The figure shows three views and two pictorial views of one solid part (mm, origin at its lowest corner). Answer the questions. A direction names the side the tool comes from. Round coordinates to 2 decimals unless told otherwise and drop trailing zeros. Write each loop counter-clockwise with the first axis right and the second up, starting at its lowest first coordinate (ties: lowest second). Pieces come first, ordered by that corner, then holes. Notation, with made-up numbers: M 51.5,7.5 L 65.5,7.5 A11 cw 65.5,22.5 Z; hole C -19.5,-4.5 d11. An arc over 180 degrees is marked long. Answer in a Markdown table with one row per item.
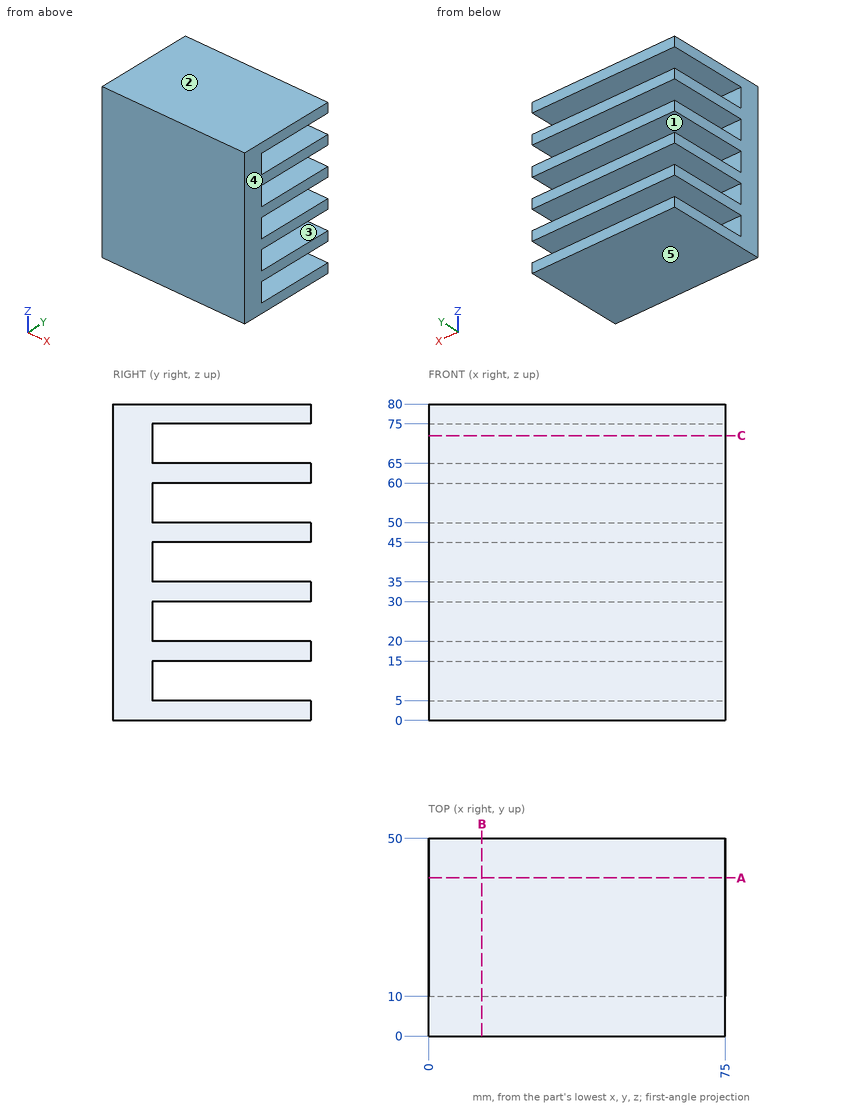
1. A tool of negligible diameter and unlimited length cuts with its end or side. For the marked faces 1 and 2, from which of +Z, -Z, +X, -X, +Y, -Y can it reach the whole face along a straight path? Write none if from no direction.
Calculated:
| item | result |
|---|---|
| face 1 | +X, -X, +Y |
| face 2 | +Z, +X, -X, +Y, -Y |
2. The part is cut by section B-B (x = 13.5). Determine the outline of the cut face in (y, z), plus the area to 3 significant figures.
Calculated:
| item | result |
|---|---|
| outline | M 0,0 L 50,0 L 50,5 L 10,5 L 10,15 L 50,15 L 50,20 L 10,20 L 10,30 L 50,30 L 50,35 L 10,35 L 10,45 L 50,45 L 50,50 L 10,50 L 10,60 L 50,60 L 50,65 L 10,65 L 10,75 L 50,75 L 50,80 L 0,80 Z |
| area | 2,000 mm² |
3. The part is cut by section C-C (z = 72). Determine the outline of the cut face in (x, y), plus the area to 3 significant figures.
Calculated:
| item | result |
|---|---|
| outline | M 0,0 L 75,0 L 75,10 L 0,10 Z |
| area | 750 mm² |
4. Determine the mould class of the marked faces 3, 4 and 5 for opening direction Z: released by +Z, released by -Z, zero draft, split by the parting line, or undercut.
Calculated:
| item | result |
|---|---|
| face 3 | undercut |
| face 4 | zero draft |
| face 5 | released by -Z |
5. Given pin 1 (8 mm diameter, centred on x = 49, z = 54.5, fed in from +Y); pin 2 (4 mm diameter, centred on x = 51.5, z = 43.5, fed in from -Y); pin 3 (1.5 mm diameter, centred on y = 15, z = 51, fed in from -X), each flat-ended and moving along its own axis, determine where each tip first touches the part or whether it passes through.
Calculated:
| item | result |
|---|---|
| pin 1 | stops at y = 10 |
| pin 2 | stops at y = 0 |
| pin 3 | passes through |
6. Consider line 1 along Z through (x, y) = (25.5, 32.5); line 2 along Y through (x, z) = (34, 58.5). Determine where each line is inside the solid, lowest interval first. Write a range as from..to.
Calculated:
| item | result |
|---|---|
| line 1 | z = 0..5, 15..20, 30..35, 45..50, 60..65, 75..80 |
| line 2 | y = 0..10 |
7. The part is cut by section A-A (y = 40). Determine the outline of the cut face in (x, z).
Calculated:
| item | result |
|---|---|
| outline | M 0,0 L 75,0 L 75,5 L 0,5 Z; M 0,15 L 75,15 L 75,20 L 0,20 Z; M 0,30 L 75,30 L 75,35 L 0,35 Z; M 0,45 L 75,45 L 75,50 L 0,50 Z; M 0,60 L 75,60 L 75,65 L 0,65 Z; M 0,75 L 75,75 L 75,80 L 0,80 Z |
